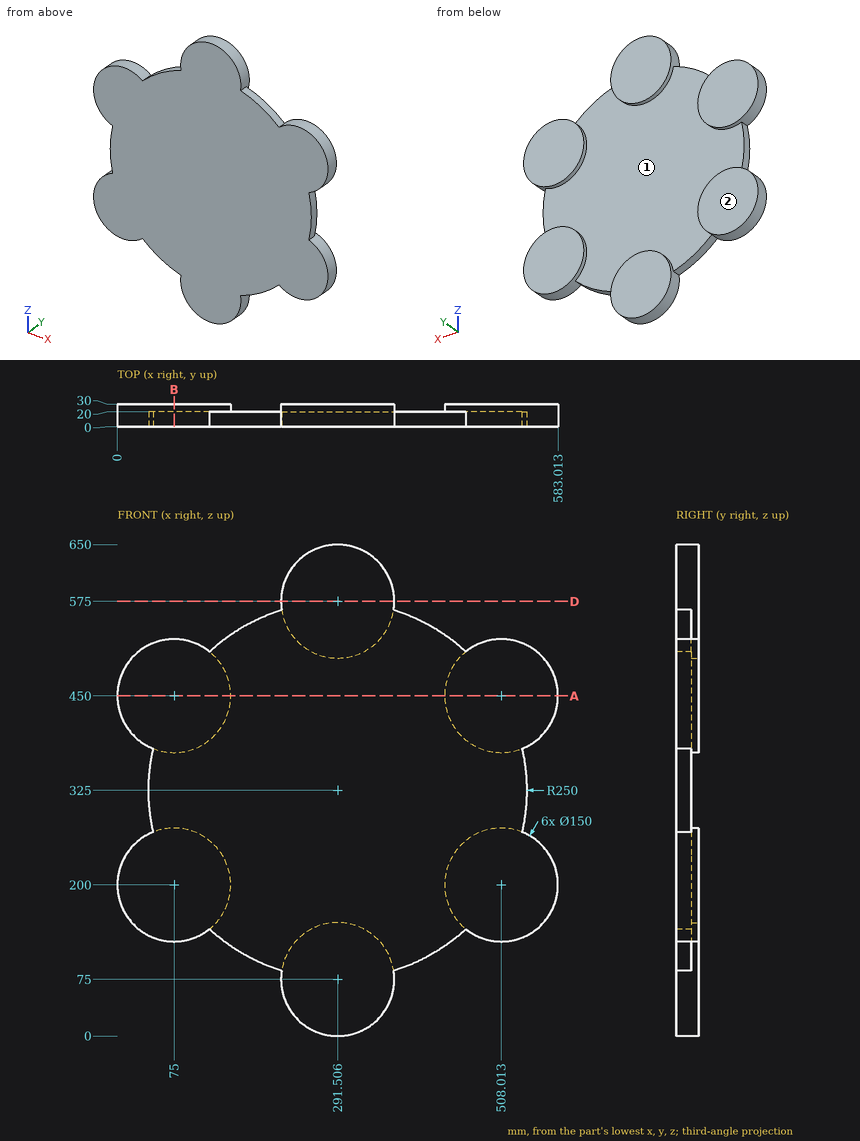
Input: dimensioned drawing with shaded views. Units: mm. Origin: part minimum x, y, z. Coordinates: 2 decimals unless noted, no trailing zeros. Order: outer loops, then holes, each group sorted by start corner. A loop starts at its lowest first (then second) coordinate and runs counter-clockwise, first axis right, second up. Notation, with made-up numbers: M 72,-16 L 97,-16 A22 cw 97,20 Z; hole C 14.25,56.25 d6. An arc over 180 degrees is marked long. Answer as CSV lines item,"result".
Q1. Line query: probe 1 along X at (y, z) = (23.75, 134) (1 decimal); probe 2 along Z at (x, y) = (264, 25.5) (1 decimal); probe 3 along X at (y, z) = (15.25, 333.5). Output: solid intervals per line, ascending. Write a range as [from, to].
Answers:
probe 1,"x = [39.4, 110.6], [245.2, 337.8], [472.4, 543.6]"
probe 2,"z = [5.2, 144.8], [505.2, 644.8]"
probe 3,"x = [41.65, 541.36]"
Q2. Draft query along Z for the marked faces 1 and 2. Return one class per face: pulls with the +Z half, pulls with the -Z half, needs draft (parallel to the pull), parting line crosses it, or undercut.
Answers:
face 1,"undercut"
face 2,"needs draft"
Q3. Section A-A on z = 450. Return the cut outline in (x, y).
Answers:
outline,"M 0,0 L 583.01,0 L 583.01,30 L 433.01,30 L 433.01,20 L 150,20 L 150,30 L 0,30 Z"
Q4. Section D-D on z = 575. Return the cut outline in (x, y).
Answers:
outline,"M 216.51,0 L 366.51,0 L 366.51,30 L 216.51,30 Z"
Q5. Section B-B on x = 75. Return the cut outline in (y, z).
Answers:
outline,"M 0,125 L 30,125 L 30,275 L 20,275 L 20,375 L 30,375 L 30,525 L 0,525 Z"
Q6. First-contact query: P1, Ø1.5, axis at y = 24, z = 487, coming from the -X side; P2, Ø3, axis at x = 410.5, y = 6, coming from the +Z side; P3, Ø1, axis at x = 306, y = 12, coming from the -Z side. Flat tips, straight axial feed; report the tip coordinate or a pass-through.
Answers:
P1,"stops at x = 9.34"
P2,"stops at z = 545.67"
P3,"stops at z = 1.32"
